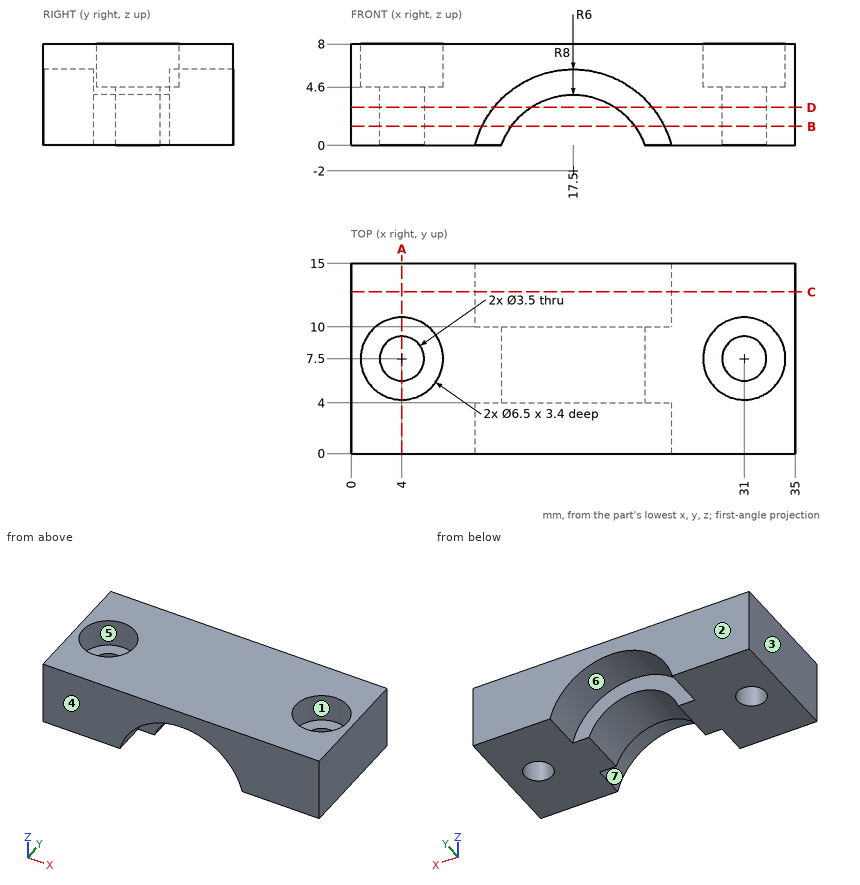
Source: three-view drawing plus pictorial views. Frame: mm from the lowest corner of the part. A direction names the side the tool comes from. Round coordinates to 2 decimals unless told otherwise and drop trailing zeros. Loops run counter-clockwise (first coordinate to the right, second up) from the corner with the lowest first, then second, coordinate; pieces in that order, holes last.
Item 1: Reachability of the marked faces 5, 6 and 7 from +Z, -Z, +X, -X, +Y, -Y: full face, straight path, thin tool, end or side. Return the list, or none.
Checked values:
face 5: +Z
face 6: -Z, +Y
face 7: -Z, -Y
Item 2: Section B-B, the plane z = 1.5. Output: boundary loops of the cut face in (x, y), plus the area to 3 significant figures.
Checked values:
outline: (0, 0) - (10.31, 0) - (10.31, 4) - (12.63, 4) - (12.63, 10) - (10.31, 10) - (10.31, 15) - (0, 15) - close; (22.37, 4) - (24.69, 4) - (24.69, 0) - (35, 0) - (35, 15) - (24.69, 15) - (24.69, 10) - (22.37, 10) - close; hole circle Ø3.5 at (4, 7.5); hole circle Ø3.5 at (31, 7.5)
area: 318 mm2
Item 3: Section A-A, the plane x = 4. Output: boundary loops of the cut face in (y, z).
Checked values:
outline: (0, 0) - (5.75, 0) - (5.75, 4.6) - (4.25, 4.6) - (4.25, 8) - (0, 8) - close; (9.25, 0) - (15, 0) - (15, 8) - (10.75, 8) - (10.75, 4.6) - (9.25, 4.6) - close
Item 4: Mould query, pull axis Y, two halves, no side actions, for the marked faces 1, 2, 3 and 4. Classes: released by +Y, released by -Y, zero draft, split by the parting line, or undercut.
Checked values:
face 1: undercut
face 2: released by +Y
face 3: zero draft
face 4: released by -Y
Item 5: Line query: L1, parallel to Y at x = 4, z = 5.7; L2, parallel to Y at x = 4, z = 3.15; L3, parallel to X at y = 9.5, z = 6.25. Output: solid intervals per line, ascending.
Checked values:
L1: y = 0 to 4.25, 10.75 to 15
L2: y = 0 to 5.75, 9.25 to 15
L3: x = 0 to 1.44, 6.56 to 28.44, 33.56 to 35
Item 6: Section C-C, the plane y = 12.75. Output: boundary loops of the cut face in (x, z), plus the area to 3 significant figures.
Checked values:
outline: (0, 0) - (9.75, 0) arc R8 cw to (25.25, 0) - (35, 0) - (35, 8) - (0, 8) - close
area: 211 mm2
Item 7: Section D-D, the plane z = 3. Output: boundary loops of the cut face in (x, y) (3 decimals), plus the area to 3 significant figures.
Checked values:
outline: (0, 0) - (11.255, 0) - (11.255, 4) - (14.183, 4) - (14.183, 10) - (11.255, 10) - (11.255, 15) - (0, 15) - close; (20.817, 4) - (23.745, 4) - (23.745, 0) - (35, 0) - (35, 15) - (23.745, 15) - (23.745, 10) - (20.817, 10) - close; hole circle Ø3.5 at (4, 7.5); hole circle Ø3.5 at (31, 7.5)
area: 354 mm2
Item 8: Contact query for a flat-ended pin moving along its axis: P1, Ø3, axis at x = 30, y = 8.5, coming from the +Z side. Output: stop coordinate, or through.
Checked values:
P1: stops at z = 4.6
